The model under review builds one solid part; all positions refer to its coordinate system, in mm. Round coordinates to 2 decimals unless told otherwise and drop trailing zeros. Order: outer loops, then holes, each group sorted by start corner. A loop starts at its lowest first (then second) coordinate and runs counter-clockwise, first axis right, second up.
from build123d import *

# Parameters (mm, degrees)
F0_W     = 45
F0_H     = 10
F1_DEPTH = 15
F2_R     = 1
F2_R_2   = 1.5
F2_R_3   = 2
F2_R_4   = 2.5
F2_R_5   = 3
F3_DEPTH = 10
F4_R     = 1
F4_R_2   = 1.5
F4_R_3   = 2
F4_R_4   = 2.5
F4_R_5   = 3
F5_DEPTH = 15


with BuildPart() as f1:
    # F0 (on Top) → F1 (new body)
    with BuildSketch(Plane.XY):
        Rectangle(F0_W, F0_H)
    extrude(amount=F1_DEPTH)

    # F2 (on face) → F3 (cut, through all)
    with BuildSketch(Plane.XZ.offset(5)):
        with Locations((-15.5, 7.5)):
            Circle(F2_R)
        with Locations((-8.5, 7.5)):
            Circle(F2_R_2)
        with Locations((-1.5, 7.5)):
            Circle(F2_R_3)
        with Locations((5.5, 7.5)):
            Circle(F2_R_4)
        with Locations((12.5, 7.5)):
            Circle(F2_R_5)
    extrude(amount=-F3_DEPTH, mode=Mode.SUBTRACT)

    # F4 (on face) → F5 (cut, through all)
    with BuildSketch(Plane.XY.offset(15)):
        with Locations((-15.5, 0)):
            Circle(F4_R)
        with Locations((-8.5, 0)):
            Circle(F4_R_2)
        with Locations((-1.5, 0)):
            Circle(F4_R_3)
        with Locations((5.5, 0)):
            Circle(F4_R_4)
        with Locations((12.5, 0)):
            Circle(F4_R_5)
    extrude(amount=-F5_DEPTH, mode=Mode.SUBTRACT)


solid = f1.part
(1) We need section B-B (y = 4). Give the boundary of the cut face in (x, z), and give its area (3 significant figures).
(2) We need section A-A (x = -8.5). Give the boundary of the cut face in (y, z), and give its area (3 significant figures).
(3) We need section D-D (x = -1.5). Give the boundary of the cut face in (y, z), and give its area (3 significant figures).
(4) We need section C-C (z = 12.25). Give the boundary of the cut face in (x, y), and give its area (3 significant figures).
(5) To check wall thickness, follow L1, parallel to X at y = 3, z = 7.5; L2, parallel to Y at x = -15.5, z = 4.25; L3, parallel to Y at x = 12.5, z = 1.5. State the ranges of each line that lie inside material, in increasing order.
(6) Clearance check with flat-ended pins moving along their axes: P1, Ø3.5, axis at x = -8.5, y = 0, coming from the +Z side; P2, Ø3, axis at x = -1.5, z = 7.5, coming from the +Y side. State where each tip first meets the part, or that it passes through.
(7) The part is to be moulded in two halves that separate along Z. For faces 1 (the cylindrical face through (-7.114, 3.021, 6.925)), 2 (the cylindrical face through (-8.695, 1.487, 12.136)), say which applies: pulls with the +Z half, pulls with the -Z half, needs draft (parallel to the pull), parting line crosses it, or undercut.
Verdict:
1. outline: (-22.5, 0) - (22.5, 0) - (22.5, 15) - (-22.5, 15) - close; hole circle Ø2 at (-15.5, 7.5); hole circle Ø3 at (-8.5, 7.5); hole circle Ø4 at (-1.5, 7.5); hole circle Ø5 at (5.5, 7.5); hole circle Ø6 at (12.5, 7.5)
1. area: 604 mm2
2. outline: (-5, 0) - (-1.5, 0) - (-1.5, 6) - (-5, 6) - close; (-5, 9) - (-1.5, 9) - (-1.5, 15) - (-5, 15) - close; (1.5, 0) - (5, 0) - (5, 6) - (1.5, 6) - close; (1.5, 9) - (5, 9) - (5, 15) - (1.5, 15) - close
2. area: 84.0 mm2
3. outline: (-5, 0) - (-2, 0) - (-2, 5.5) - (-5, 5.5) - close; (-5, 9.5) - (-2, 9.5) - (-2, 15) - (-5, 15) - close; (2, 0) - (5, 0) - (5, 5.5) - (2, 5.5) - close; (2, 9.5) - (5, 9.5) - (5, 15) - (2, 15) - close
3. area: 66.0 mm2
4. outline: (-22.5, -5) - (22.5, -5) - (22.5, 5) - (-22.5, 5) - close; hole circle Ø2 at (-15.5, 0); hole circle Ø3 at (-8.5, 0); hole circle Ø4 at (-1.5, 0); hole circle Ø5 at (5.5, 0); hole circle Ø6 at (12.5, 0)
4. area: 379 mm2
5. L1: x = -22.5 to -16.5, -14.5 to -10, -7 to -3.5, 0.5 to 3, 8 to 9.5, 15.5 to 22.5
5. L2: y = -5 to -1, 1 to 5
5. L3: y = -5 to -3, 3 to 5
6. P1: stops at z = 15
6. P2: passes through
7. face 1: undercut
7. face 2: needs draft
